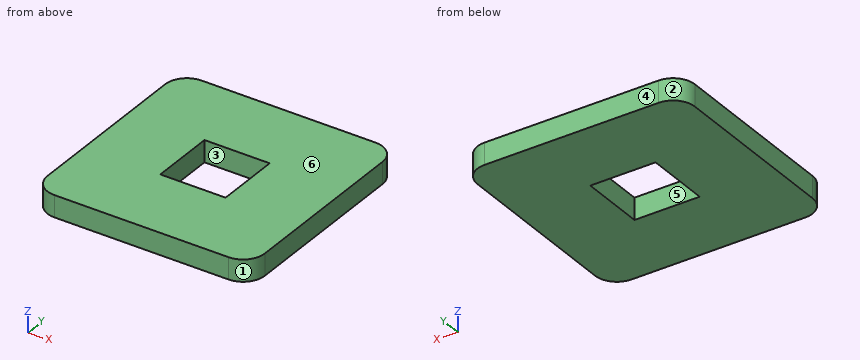
Autodesk Inventor part; units mm, degrees
ref_plane "YZ Plane" through (0, 0, 0) normal (1, 0, 0) x (0, 1, 0)
ref_plane "XZ Plane" through (0, 0, 0) normal (0, 1, 0) x (-1, 0, 0)
ref_plane "XY Plane" through (0, 0, 0) normal (0, 0, 1) x (1, 0, 0)
sketch "Esboço1" plane through (0, 0, 0) normal (0, 0, 1) x (1, 0, 0)
  line L0 (-50, -50) -> (50, -50)
  line L1 (50, -50) -> (50, 50)
  line L2 (50, 50) -> (-50, 50)
  line L3 (-50, 50) -> (-50, -50)
  line L4 (-50, -50) -> (50, 50) construction
  line L5 (50, -50) -> (-50, 50) construction
  line L6 (-15, -15) -> (15, -15)
  line L7 (15, -15) -> (15, 15)
  line L8 (15, 15) -> (-15, 15)
  line L9 (-15, 15) -> (-15, -15)
  line L10 (-15, -15) -> (15, 15) construction
  line L11 (15, -15) -> (-15, 15) construction
  point P0 (0, 0)
  dimension "d0" = 100
  dimension "d1" = 100
  dimension "d2" = 30
  dimension "d3" = 30
extrude "Extrusão1" add sketch "Esboço1" along normal blind 10
fillet "Arredondamento1" radius 10 1 edges at (50, 50, 5)
fillet "Arredondamento2" radius 10 1 edges at (-50, 50, 5)
fillet "Arredondamento3" radius 10 1 edges at (50, -50, 5)
fillet "Arredondamento4" radius 10 1 edges at (-50, -50, 5)
properties part number "placa_furo_quadrado"
Build history of the part. All positions in model axes, mm. Face numbers are marked on the shaded views. A direction names the side the tool comes from. Give positions to 0.01 mm unless a question says otherwise; leave off trailing zeros. Loops run counter-clockwise (first coordinate to the right, second up) from the corner with the lowest first, then second, coordinate; pieces in that order, holes last.
Item 1: Slice it at A-A, the plane x = -8. List the corners of the cut face in (y, z), and give its area (3 significant figures).
Answers follow:
outline: (-50, 0) - (-15, 0) - (-15, 10) - (-50, 10) - close; (15, 0) - (50, 0) - (50, 10) - (15, 10) - close
area: 700 mm2
Item 2: Which spindle directions (+Z, -Z, +X, -X, +Y, -Y) get a long thin tool onto all of the face, cutting with end or side? Do the marked faces 5 and 6. Say none if no direction does.
Answers follow:
face 5: +Z, -Z
face 6: +Z, +X, -X, +Y, -Y
Item 3: Slice it at C-C, the plane z = 3.75. List the corners of the cut face in (x, y), and give its area (3 significant figures).
Answers follow:
outline: (-50, -40) arc R10 ccw to (-40, -50) - (40, -50) arc R10 ccw to (50, -40) - (50, 40) arc R10 ccw to (40, 50) - (-40, 50) arc R10 ccw to (-50, 40) - close; hole (-15, -15) - (15, -15) - (15, 15) - (-15, 15) - close
area: 9,010 mm2
Item 4: Pull direction X, two halves, no side cores. Call the marked faces 1, 2, 3 and 4: released by +X, released by -X, zero draft, split by the parting line, or undercut.
Answers follow:
face 1: released by +X
face 2: released by -X
face 3: undercut
face 4: zero draft
Item 5: Drill centre lines: line 1 (X direction, y = -13, z = 6.75); line 2 (X direction, y = 42, z = 2.25). Where is each one in solid material? Low to high.
Answers follow:
line 1: x = -50 to -15, 15 to 50
line 2: x = -49.8 to 49.8
Item 6: Slice it at D-D, the plane x = -44. List the corners of the cut face in (y, z).
Answers follow:
outline: (-49.17, 0) - (49.17, 0) - (49.17, 10) - (-49.17, 10) - close
